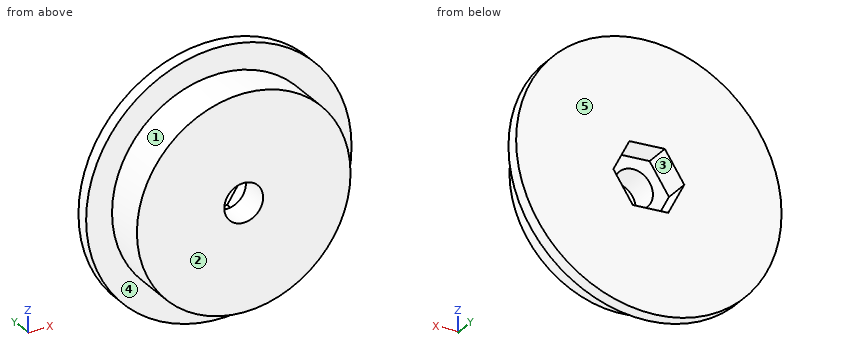
```python
from build123d import *

# Parameters (mm, degrees)
F0_R     = 41
F0_R_2   = 33
F2_DEPTH = 4
F1_R     = 33
F1_R_2   = 6
F3_DEPTH = 17
F4_R     = 6
F5_DEPTH = 8


with BuildPart() as f2:
    # F0 (on Front) → F2 (new body)
    with BuildSketch(Plane.XZ):
        Circle(F0_R)
        Circle(F0_R_2, mode=Mode.SUBTRACT)
    extrude(amount=F2_DEPTH)

    # F1 (on Front) → F3 (join)
    with BuildSketch(Plane.XZ):
        Circle(F1_R)
        Circle(F1_R_2, mode=Mode.SUBTRACT)
    extrude(amount=F3_DEPTH)

    # F4 (on Front) → F5 (cut)
    with BuildSketch(Plane.XZ):
        Polygon((-10.952806, 0.607765), (-6.002742, -9.181526), (4.950063, -9.78929), (10.952806, -0.607765), (6.002742, 9.181526), (-4.950063, 9.78929), align=None)
        Circle(F4_R, mode=Mode.SUBTRACT)
    extrude(amount=F5_DEPTH, mode=Mode.SUBTRACT)


solid = f2.part
```
Part model, mm, in its own coordinate system. Face numbers are marked on the shaded views. A direction names the side the tool comes from. Round coordinates to 2 decimals unless told otherwise and drop trailing zeros. Order: outer loops, then holes, each group sorted by start corner. A loop starts at its lowest first (then second) coordinate and runs counter-clockwise, first axis right, second up. Notation, with made-up numbers: M 14.25,-14.75 L 54.25,-14.75 A8 ccw 54.25,-5.75 Z; hole C 55,14.5 d9. An arc over 180 degrees is marked long. Answer in a Markdown table with one row per item. Add a question column.
Q1. Cut at C-C on x = 24. Give the cut face in (y, z), and give its area (3 significant figures).
Q2. Wall check: L1, parallel to Z at x = 0, y = -12.5; L2, parallel to Z at x = -1.5, y = -4.25; L3, parallel to Y at x = 23.5, z = -27. Give the ranges that are in metal, low to high. Write a range as from..to.
Q3. Cut at D-D on y = -11. Give the cut face in (x, z).
Q4. Pin check, flat tips, straight feed: pin 1 (6 mm diameter, centred on y = -5, z = -11.5, fed in from -X); pin 2 (6 mm diameter, centred on x = 0, y = -2.5, fed in from -Z); pin 3 (4 mm diameter, centred on x = -6.5, y = -10, fed in from -Z). Stop position of each tip, or through.
Q5. Mould opens along X. For the marked faces 1, 2 and 3 say: +X half, -X half, draft (parallel to the pull), parting line (faces both ways), or undercut.
Q6. Cut at B-B on x = 0. Give the cut face in (y, z).
Q7. 3-axis set-ups, long thin cutter, end or side, ignore diameter. For the marked faces 4 and 5: which of +Z, -Z, +X, -X, +Y, -Y reach the whole face in a straight line?
Q8. Cut at A-A on y = -2.75. Give the cut face in (x, z).
Established:
| question | item | result |
|---|---|---|
| 1 | outline | M -17,-22.65 L -4,-22.65 L -4,-33.24 L 0,-33.24 L 0,33.24 L -4,33.24 L -4,22.65 L -17,22.65 Z |
| 1 | area | 855 mm2 |
| 2 | L1 | z = -33..-6, 6..33 |
| 2 | L2 | z = -32.97..-9.43, 9.6..32.97 |
| 2 | L3 | y = -4..0 |
| 3 | outline | C 0,0 d66; hole C 0,0 d12 |
| 4 | pin 1 | stops at x = -40.07 |
| 4 | pin 2 | stops at z = -41 |
| 4 | pin 3 | stops at z = -32.69 |
| 5 | face 1 | parting line |
| 5 | face 2 | draft |
| 5 | face 3 | undercut |
| 6 | outline | M -17,-33 L -4,-33 L -4,-41 L 0,-41 L 0,-9.51 L -8,-9.51 L -8,-6 L -17,-6 Z; M -17,6 L -8,6 L -8,9.51 L 0,9.51 L 0,41 L -4,41 L -4,33 L -17,33 Z |
| 7 | face 4 | -Y |
| 7 | face 5 | +Z, -Z, +X, -X, +Y |
| 8 | outline | C 0,0 d82; hole M -10.95,0.61 L -6,-9.18 L 4.95,-9.79 L 10.95,-0.61 L 6,9.18 L -4.95,9.79 Z |
